Input: part model. Units: mm. Frame: model coordinates. Face numbers are marked on the shaded views. A direction names the side the tool comes from. Coordinates: 2 decimals unless noted, no trailing zeros. Loops run counter-clockwise (first coordinate to the right, second up) from the corner with the lowest first, then second, coordinate; pieces in that order, holes last. Notation, with made-up numbers: M -21,-21 L 7,-21 A14 ccw 7,2 Z; hole C 49,-24 d2. An arc over 180 degrees is marked long. Use a Markdown table: item, result. Add a question column.
1. Set-up query: the marked faces 4 and 5. Return all of +Z, -Z, +X, -X, +Y, -Y with unobstructed straight access to the full face (end or side cutting, diameter ignored); none if empty.
2. Section D-D on y = 2.75. Output: boundary loops of the cut face in (x, z).
3. Line query: L1, parallel to X at y = 6.55, z = 0; L2, parallel to X at y = 1, z = -3.5; L3, parallel to Y at x = 3.25, z = 2.25. Output: solid intervals per line, ascending. Write a range as [from, to].
4. Section B-B on y = 6.25. Output: boundary loops of the cut face in (x, z), then the cut area to 3 significant figures.
5. Section A-A on x = 0. Output: boundary loops of the cut face in (y, z), then the cut area to 3 significant figures.
6. Draft query along X for the marked faces 1, 2 and 3. Return one class per face: +X half, -X half, draft (parallel to the pull), parting line (faces both ways), or undercut.
7. Section C-C on z = 0. Output: boundary loops of the cut face in (x, y), then the cut area to 3 significant figures.
```python
from build123d import *

# Parameters (mm, degrees)
SKETCH1_W           = 20
SKETCH1_H           = 9.6
BOSS_EXTRUDE1_DEPTH = 5
SKETCH2_W           = 20
SKETCH2_H           = 9.6
SKETCH2_R           = 2.5
BOSS_EXTRUDE2_DEPTH = 2.5
FILLET1_R           = 1


with BuildPart() as part:
    # Sketch1 → Boss-Extrude1 (new body)
    with BuildSketch(Plane(origin=(0, 0, 0), x_dir=(1, 0, 0), z_dir=(0, 1, 0))):
        Rectangle(SKETCH1_W, SKETCH1_H)
        Polygon((4.618802154, 0), (2.309401077, 4), (-2.309401077, 4), (-4.618802154, 0), (-2.309401077, -4), (2.309401077, -4), align=None, mode=Mode.SUBTRACT)
    extrude(amount=BOSS_EXTRUDE1_DEPTH)

    # Sketch2 → Boss-Extrude2 (add)
    with BuildSketch(Plane(origin=(0, 5, 0), x_dir=(1, 0, 0), z_dir=(0, 1, 0))):
        Rectangle(SKETCH2_W, SKETCH2_H)
        with Locations(Location((0, 0, 0), (0, 0, 270))):
            Circle(SKETCH2_R, mode=Mode.SUBTRACT)
    extrude(amount=BOSS_EXTRUDE2_DEPTH)

    # Fillet1
    fillet1_edges = [part.edges().sort_by_distance(p)[0] for p in [
        (2.309401077, 2.5, 4),
        (4.618802154, 2.5, 0),
        (2.309401077, 2.5, -4),
        (-2.309401077, 2.5, -4),
        (-4.618802154, 2.5, 0),
        (-2.309401077, 2.5, 4),
        (10, 3.75, 4.8),
        (-10, 3.75, 4.8),
        (-10, 3.75, -4.8),
        (10, 3.75, -4.8),
    ]]
    fillet(fillet1_edges, radius=FILLET1_R)


solid = part.part
```
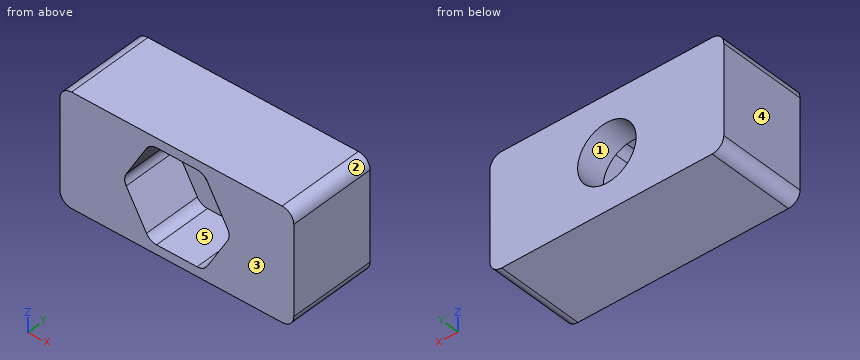
Answers below:
| question | item | result |
|---|---|---|
| 1 | face 4 | +Z, -Z, -X, +Y, -Y |
| 1 | face 5 | -Y |
| 2 | outline | M -10,-3.8 A1 ccw -9,-4.8 L 9,-4.8 A1 ccw 10,-3.8 L 10,3.8 A1 ccw 9,4.8 L -9,4.8 A1 ccw -10,3.8 Z; hole M -4.33,-0.5 L -2.6,-3.5 A1 ccw -1.73,-4 L 1.73,-4 A1 ccw 2.6,-3.5 L 4.33,-0.5 A1 ccw 4.33,0.5 L 2.6,3.5 A1 ccw 1.73,4 L -1.73,4 A1 ccw -2.6,3.5 L -4.33,0.5 A1 ccw Z |
| 3 | L1 | x = [-10, -2.5], [2.5, 10] |
| 3 | L2 | x = [-10, -2.6], [2.6, 10] |
| 3 | L3 | y = [5, 7.5] |
| 4 | outline | M -10,-3.8 A1 ccw -9,-4.8 L 9,-4.8 A1 ccw 10,-3.8 L 10,3.8 A1 ccw 9,4.8 L -9,4.8 A1 ccw -10,3.8 Z; hole C 0,0 d5 |
| 4 | area | 172 mm² |
| 5 | outline | M 0,-4.8 L 7.5,-4.8 L 7.5,-2.5 L 5,-2.5 L 5,-4 L 0,-4 Z; M 0,4 L 5,4 L 5,2.5 L 7.5,2.5 L 7.5,4.8 L 0,4.8 Z |
| 5 | area | 19.5 mm² |
| 6 | face 1 | undercut |
| 6 | face 2 | +X half |
| 6 | face 3 | draft |
| 7 | outline | M -10,0 L -4.46,0 L -4.46,5 L -2.5,5 L -2.5,7.5 L -10,7.5 Z; M 2.5,5 L 4.46,5 L 4.46,0 L 10,0 L 10,7.5 L 2.5,7.5 Z |
| 7 | area | 92.9 mm² |
